Answer from the drawing. Dimensions are ordinates in mm from the lowest x, y and z of the part. Give positions to 0.01 mm unless a question says otherwise; leave off trailing zeros. Order: outer loops, then holes, each group sorted by start corner. A loop starts at its lowest first (then second) coordinate and runs counter-clockwise, first axis right, second up.
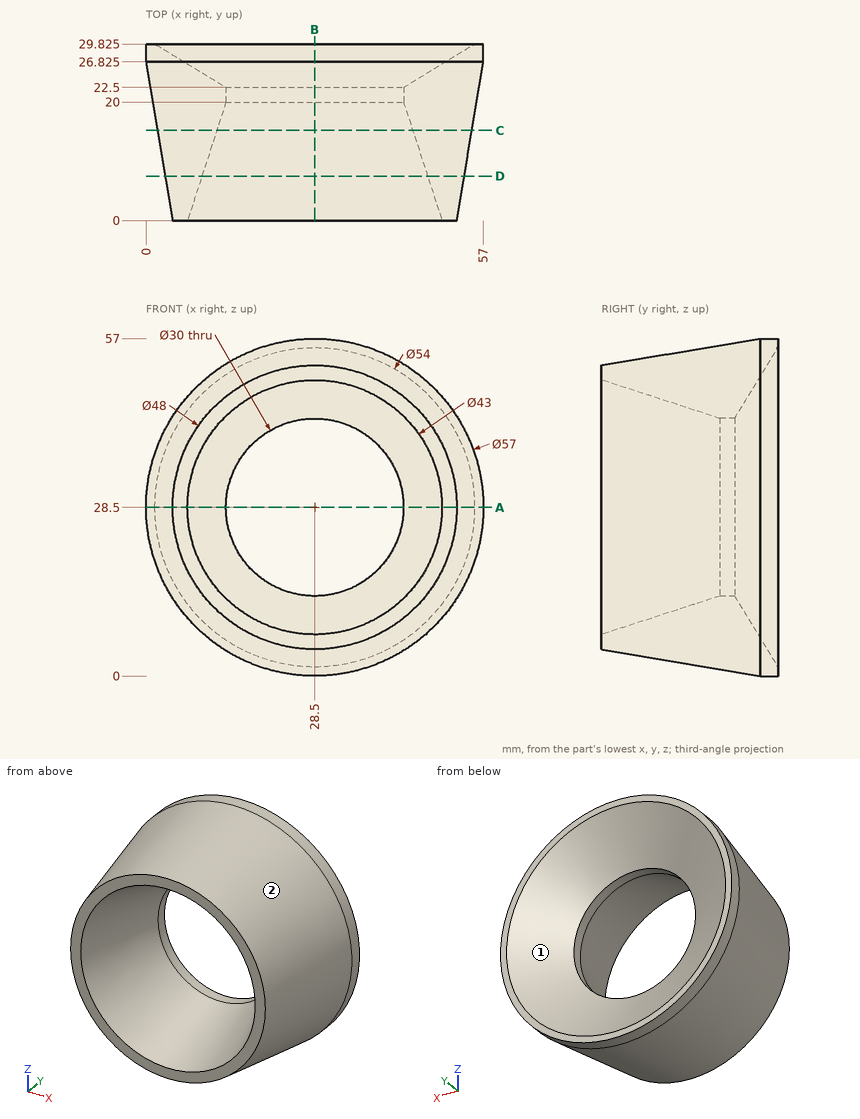
1. The part is cut by section B-B (x = 28.5). Write down the section's boundary in (y, z) (1 decimal).
Findings below:
outline: (0, 4.5) - (26.8, 0) - (29.8, 0) - (29.8, 1.5) - (22.5, 13.5) - (20, 13.5) - (0, 7) - close; (0, 50) - (20, 43.5) - (22.5, 43.5) - (29.8, 55.5) - (29.8, 57) - (26.8, 57) - (0, 52.5) - close
2. The part is cut by section C-C (y = 15.25). Write down the section's boundary in (x, z), then the cut area to 3 significant figures.
Findings below:
outline: circle Ø53.12 at (28.5, 28.5); hole circle Ø33.09 at (28.5, 28.5)
area: 1,360 mm2
3. The part is cut by section D-D (y = 7.5). Write down the section's boundary in (x, z) (1 decimal).
Findings below:
outline: circle Ø50.5 at (28.5, 28.5); hole circle Ø38.1 at (28.5, 28.5)
4. The mould has two halves that part along Z. Classify the marked faces 1 and 2: pulls with the +Z half, pulls with the -Z half, needs draft (parallel to the pull), parting line crosses it, or undercut.
Findings below:
face 1: undercut
face 2: parting line crosses it
5. The part is cut by section A-A (z = 28.5). Write down the section's boundary in (x, y) (1 decimal).
Findings below:
outline: (0, 26.8) - (4.5, 0) - (7, 0) - (13.5, 20) - (13.5, 22.5) - (1.5, 29.8) - (0, 29.8) - close; (43.5, 20) - (50, 0) - (52.5, 0) - (57, 26.8) - (57, 29.8) - (55.5, 29.8) - (43.5, 22.5) - close
6. Straight lines are drawn through the part: probe 1 along Z at (x, y) = (27, 9.5); probe 2 along X at (y, z) = (16, 29.5) (1 decimal); probe 3 along Z at (x, y) = (28.5, 21.3). For each, find the intervals that lie inside material, in ascending order.
Findings below:
probe 1: z = 2.95 to 10.15, 46.85 to 54.05
probe 2: x = 1.8 to 12.2, 44.8 to 55.2
probe 3: z = 0.93 to 13.5, 43.5 to 56.07
7. Given P1, Ø3, axis at x = 46.5, y = 12, coming from the -Z side; P2, Ø2, axis at x = 25, y = 4.5, coming from the -Z side; P3, Ø12, axis at x = 27, y = 8.5, coming from the -Z side, each flat-ended and moving along its own axis, determine where each tip first touches the part or whether it passes through.
Findings below:
P1: stops at z = 8.35
P2: stops at z = 3.78
P3: stops at z = 2.09
